```python
from build123d import *

# Parameters (mm, degrees)
SKETCH1_W           = 90
SKETCH1_H           = 60
BOSS_EXTRUDE1_DEPTH = 20
CUT_EXTRUDE1_DEPTH  = 61
SKETCH3_R           = 4.3
CUT_EXTRUDE2_DEPTH  = 21
CHAMFER1_SIZE       = 1
CHAMFER2_SIZE       = 1


with BuildPart() as part:
    # Sketch1 → Boss-Extrude1 (new body)
    with BuildSketch(Plane(origin=(0, 0, 0), x_dir=(1, 0, 0), z_dir=(0, 1, 0))):
        Rectangle(SKETCH1_W, SKETCH1_H)
    extrude(amount=BOSS_EXTRUDE1_DEPTH)

    # Sketch2 → Cut-Extrude1 (cut, through all)
    with BuildSketch(Plane.XY.offset(30)):
        Polygon((28, 24.25), (-28, 24.25), (-28, 15.75), (-7.8, 15.75), (-7.8, 20), (7.8, 20), (7.8, 15.75), (28, 15.75), align=None)
    extrude(amount=-CUT_EXTRUDE1_DEPTH, mode=Mode.SUBTRACT)

    # Sketch3 → Cut-Extrude2 (cut, through all)
    with BuildSketch(Plane.XZ):
        with Locations((-35, 15)):
            Circle(SKETCH3_R)
        with Locations((-35, -15)):
            Circle(SKETCH3_R)
        with Locations((35, -14.217273236)):
            Circle(SKETCH3_R)
        with Locations((35, 15)):
            Circle(SKETCH3_R)
    extrude(amount=-CUT_EXTRUDE2_DEPTH, mode=Mode.SUBTRACT)

    # Chamfer1
    chamfer1_edges = [part.edges().sort_by_distance(p)[0] for p in [
        (28, 20, 0),
        (-28, 20, 0),
        (7.8, 20, 0),
        (-7.8, 20, 0),
    ]]
    chamfer(chamfer1_edges, length=CHAMFER1_SIZE)

    # Chamfer2
    chamfer2_edges = [part.edges().sort_by_distance(p)[0] for p in [
        (-39.3, 20, 15),
        (-39.3, 20, -15),
        (30.7, 20, -14.217273236),
        (30.7, 20, 15),
    ]]
    chamfer(chamfer2_edges, length=CHAMFER2_SIZE)


solid = part.part
```
Geometry: final body of the model. Coordinates: model frame, mm. A direction names the side the tool comes from. Give positions to 0.01 mm unless a question says otherwise; leave off trailing zeros. Order: outer loops, then holes, each group sorted by start corner. A loop starts at its lowest first (then second) coordinate and runs counter-clockwise, first axis right, second up. Notation, with made-up numbers: M 50.25,56 L 78.25,56 A23 ccw 78.25,65 Z; hole C -26,38.25 d3. An arc over 180 degrees is marked long. Answer as CSV lines item,"result". Start each with the question number.
1) Line query: line 1 (Z direction, x = 35, y = 8.75); line 2 (Z direction, x = -35, y = 11); line 3 (X direction, y = 1.25, z = -16). Output: solid intervals per line, ascending. Write a range as from..to.
2) Cut plane C-C (x = -35). Output: boundary loops of the cut face in (y, z).
3) First-contact query: P1, Ø7.5, axis at x = 35, z = 15, coming from the +Y side; P2, Ø10, axis at x = 20.5, z = 14, coming from the +Y side. Flat tips, straight axial feed; report the tip coordinate or a pass-through.
4) Cut plane B-B (z = 15). Output: boundary loops of the cut face in (x, y), then the cut area to 3 significant figures.
5) Cut plane D-D (z = 0.5). Output: boundary loops of the cut face in (x, y), then the cut area to 3 significant figures.
6) Set-up query: faces 4 (the cylindrical face through (34.44, 9.367, 19.263)), 5 (the flat face through (-18, 15.75, 0)). Return all of +Z, -Z, +X, -X, +Y, -Y with unobstructed straight access to the full face (end or side cutting, diameter ignored); none if empty.
7) Mould query, pull axis X, two halves, no side actions, for faces 1 (the flat face through (-45, 10, 0)), 2 (the flat face through (7.8, 17, 0)), 3 (the flat face through (-1, 10, -30)). Classes: +X half, -X half, draft (parallel to the pull), parting line (faces both ways), or undercut.
8) Cut plane A-A (y = 18). Output: boundary loops of the cut face in (x, z).
Findings below:
1,line 1,"z = -30..-18.52, -9.92..10.7, 19.3..30"
1,line 2,"z = -30..-19.3, -10.7..10.7, 19.3..30"
1,line 3,"x = -45..-39.18, -30.82..31.09, 38.91..45"
2,outline,"M 0,-30 L 20,-30 L 20,-20.3 L 19,-19.3 L 0,-19.3 Z; M 0,-10.7 L 19,-10.7 L 20,-9.7 L 20,9.7 L 19,10.7 L 0,10.7 Z; M 0,19.3 L 19,19.3 L 20,20.3 L 20,30 L 0,30 Z"
3,P1,"passes through"
3,P2,"stops at y = 15.75"
4,outline,"M -45,0 L -39.3,0 L -39.3,19 L -40.3,20 L -45,20 Z; M -30.7,0 L 30.7,0 L 30.7,19 L 29.7,20 L 29,20 L 28,19 L 28,15.75 L 7.8,15.75 L 7.8,19 L 6.8,20 L -6.8,20 L -7.8,19 L -7.8,15.75 L -28,15.75 L -28,19 L -29,20 L -29.7,20 L -30.7,19 Z; M 39.3,0 L 45,0 L 45,20 L 40.3,20 L 39.3,19 Z"
4,area,"1,280 mm²"
5,outline,"M -45,0 L 45,0 L 45,20 L 29,20 L 28,19 L 28,15.75 L 7.8,15.75 L 7.8,19 L 6.8,20 L -6.8,20 L -7.8,19 L -7.8,15.75 L -28,15.75 L -28,19 L -29,20 L -45,20 Z"
5,area,"1,630 mm²"
6,face 4,"+Y, -Y"
6,face 5,"+Z, -Z, +Y"
7,face 1,"-X half"
7,face 2,"undercut"
7,face 3,"draft"
8,outline,"M -45,-30 L -28,-30 L -28,30 L -45,30 Z; M -7.8,-30 L 7.8,-30 L 7.8,30 L -7.8,30 Z; M 28,-30 L 45,-30 L 45,30 L 28,30 Z; hole C -35,-15 d8.6; hole C -35,15 d8.6; hole C 35,-14.22 d8.6; hole C 35,15 d8.6"
